from build123d import *

# Parameters (mm, degrees)
SKETCH1_R           = 3
BOSS_EXTRUDE1_DEPTH = 5


with BuildPart() as part:
    # Sketch1 → Boss-Extrude1 (new body)
    with BuildSketch(Plane.XY):
        with BuildLine():
            Line((-39, -63.5), (39, -63.5))
            ThreePointArc((39, -63.5), (42.535533906, -62.035533906), (44, -58.5))
            Line((44, -58.5), (44, 58.5))
            ThreePointArc((44, 58.5), (42.535533906, 62.035533906), (39, 63.5))
            Line((39, 63.5), (-39, 63.5))
            ThreePointArc((-39, 63.5), (-42.535533906, 62.035533906), (-44, 58.5))
            Line((-44, 58.5), (-44, -58.5))
            ThreePointArc((-44, -58.5), (-42.535533906, -62.035533906), (-39, -63.5))
        make_face()
        with Locations((-30, 40)):
            Circle(SKETCH1_R, mode=Mode.SUBTRACT)
        with Locations((30, 40)):
            Circle(SKETCH1_R, mode=Mode.SUBTRACT)
        Circle(SKETCH1_R, mode=Mode.SUBTRACT)
        with BuildLine():
            Line((27, -30), (27, -50))
            ThreePointArc((27, -50), (30, -53), (33, -50))
            Line((33, -50), (33, -30))
            ThreePointArc((33, -30), (30, -27), (27, -30))
        make_face(mode=Mode.SUBTRACT)
        with BuildLine():
            Line((-33, -30), (-33, -50))
            ThreePointArc((-33, -50), (-30, -53), (-27, -50))
            Line((-27, -50), (-27, -30))
            ThreePointArc((-27, -30), (-30, -27), (-33, -30))
        make_face(mode=Mode.SUBTRACT)
    extrude(amount=BOSS_EXTRUDE1_DEPTH)


solid = part.part
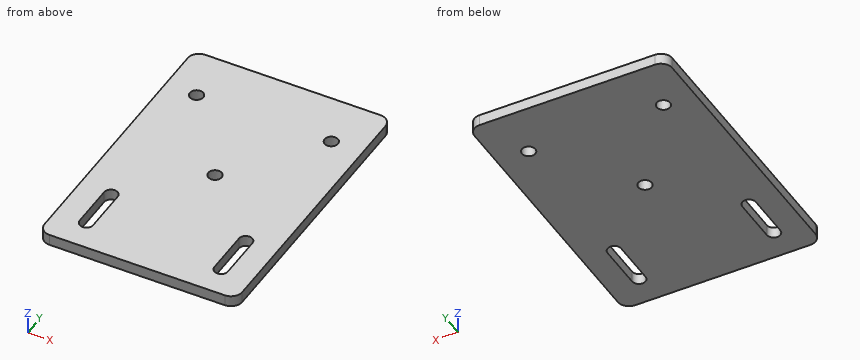
Here's how the part is built. I have some questions about the finished solid (model axes, mm). Round coordinates to 2 decimals unless told otherwise and drop trailing zeros. Loops run counter-clockwise (first coordinate to the right, second up) from the corner with the lowest first, then second, coordinate; pieces in that order, holes last. Notation, with made-up numbers: M 84.5,30 L 91.5,30 A29 cw 91.5,60 Z; hole C 61.25,38.5 d1. An arc over 180 degrees is marked long. Write each question's results on one line, items separated by ' | '. Start each with the question number.
(1) I want a section at B-B (y = -47.5). Please give me the cut outline in (x, z), then the cut area to 3 significant figures.
(2) I want a section at C-C (z = 1.95). Please give me the cut outline in (x, y).
(3) If I drill on probe 1 along Y at (x, z) = (-30, 1.45); probe 2 along X at (y, z) = (-45, 0.2); probe 3 along X at (y, z) = (1.5, 0.45), over which ranges is the centre line in solid material (lowest first)? Write a range as from..to.
(4) I want a section at A-A (x = 30). Please give me the cut outline in (y, z), then the cut area to 3 significant figures.
(5) Will this pin go through, and if not, where does the flat tip stop? P1, Ø3.5, axis at x = 30, y = 40, coming from the -Z side.
Solved:
1) outline: M -44,0 L -33,0 L -33,5 L -44,5 Z; M -27,0 L 27,0 L 27,5 L -27,5 Z; M 33,0 L 44,0 L 44,5 L 33,5 Z | area: 380 mm²
2) outline: M -44,-58.5 A5 ccw -39,-63.5 L 39,-63.5 A5 ccw 44,-58.5 L 44,58.5 A5 ccw 39,63.5 L -39,63.5 A5 ccw -44,58.5 Z; hole M -33,-50 A3 ccw -27,-50 L -27,-30 A3 ccw -33,-30 Z; hole C -30,40 d6; hole C 0,0 d6; hole M 27,-50 A3 ccw 33,-50 L 33,-30 A3 ccw 27,-30 Z; hole C 30,40 d6
3) probe 1: y = -63.5..-53, -27..37, 43..63.5 | probe 2: x = -44..-33, -27..27, 33..44 | probe 3: x = -44..-2.6, 2.6..44
4) outline: M -63.5,0 L -53,0 L -53,5 L -63.5,5 Z; M -27,0 L 37,0 L 37,5 L -27,5 Z; M 43,0 L 63.5,0 L 63.5,5 L 43,5 Z | area: 475 mm²
5) P1: passes through
